The listing builds one solid part. Answer for the finished solid, in the listing's coordinates (mm). Face numbers are marked on the shaded views. A direction names the side the tool comes from. Coordinates: 2 decimals unless noted, no trailing zeros. Write each loop counter-clockwise with the first axis right and the second up, starting at its lowest first coordinate (ties: lowest second). Pieces come first, ordered by that corner, then holes.
(1) The part is cut by section C-C on y = 14.5. Determine the outline of the cut face in (x, z), plus the area to 3 significant figures.
(2) The part is cut by section A-A on z = 25. Determine the outline of the cut face in (x, y).
(3) The part is cut by section D-D on z = 17.5. Determine the outline of the cut face in (x, y).
(4) For a pull along Y with two mould halves and no side action, classify the marked faces 6, 7, 8 and 9 as +Y half, -Y half, draft (parallel to the pull), parting line (faces both ways), or undercut.
(5) The part is cut by section B-B on x = 7. Determine the outline of the cut face in (y, z).
(6) Given P1, Ø2.5, axis at x = 39.57, z = 25, coming from the +Y side; P2, Ø7.5, axis at y = -26.5, z = 4, coming from the +X side; P3, Ø3, axis at x = 3, y = -28, coming from the +Z side; P4, Ø3, axis at y = -7.5, z = 24.5, coming from the -X side, each flat-ended and moving along its own axis, determine where each tip first touches the part or whether it passes through.
(7) Which of the six approach directions +Z, -Z, +X, -X, +Y, -Y give full straight-line access (tool end or side, diameter ignored) to the marked faces 1, 2, 3, 4 and 5?
(8) Straight lines are drawn through the part: line 1 (X direction, y = -5, z = 25); line 2 (Y direction, x = 39, z = 11); line 3 (X direction, y = -7, z = 17). For each, find the intervals that lie inside material, in ascending order.
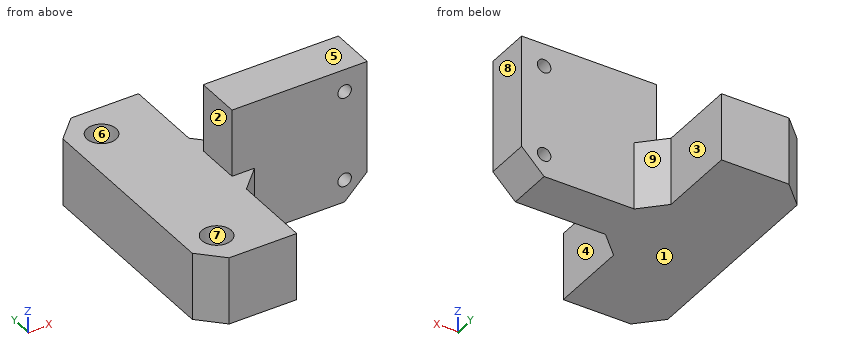
Autodesk Inventor part; units mm, degrees
ref_plane "YZ Plane" through (0, 0, 0) normal (1, 0, 0) x (0, 1, 0)
ref_plane "XZ Plane" through (0, 0, 0) normal (0, 1, 0) x (-1, 0, 0)
ref_plane "XY Plane" through (0, 0, 0) normal (0, 0, 1) x (1, 0, 0)
sketch "Sketch1" plane through (0, 0, 0) normal (0, 0, 1) x (1, 0, 0)
  line L0 (-5.4307, 20.6828) -> (14.5693, 20.6828)
  line L1 (14.5693, 20.6828) -> (14.5693, -34.3172)
  line L2 (14.5693, -34.3172) -> (-5.4307, -34.3172)
  line L3 (-5.4307, -34.3172) -> (-5.4307, 20.6828)
  point P0 (0, 0)
  dimension "d0" = 55
  dimension "d1" = 20
extrude "Extrusion1" add sketch "Sketch1" along normal blind 15
sketch "Sketch2" plane through (0, 0, 15) normal (0, 0, 1) x (1, 0, 0)
  line L0 (14.5693, 20.6828) -> (-5.4307, 20.6828)
  line L1 (-5.4307, -34.3172) -> (-5.4307, 20.6828)
  line L2 (-5.4307, -34.3172) -> (14.5693, -34.3172)
  circle A0 centre (1.5693, 13.1828) radius 3.25
  circle A1 centre (1.5693, -26.8172) radius 3.25
  point P0 (0, 0)
  dimension "d4" = 40
  dimension "d5" = 7.5
  dimension "d6" = 7
  dimension "d7" = 7.5
  dimension "d8" = 6.5
  dimension "d9" = 6.5
extrude "Extrusion2" cut sketch "Sketch2" against normal blind 10
sketch "Sketch3" plane through (0, 0, 0) normal (0, 0, -1) x (-1, 0, 0)
  line L0 (-14.5693, -34.3172) -> (-14.5693, 20.6828)
  line L1 (-14.5693, -1.8172) -> (-44.5693, -1.8172)
  line L2 (-44.5693, -1.8172) -> (-44.5693, -11.8172)
  line L3 (-44.5693, -11.8172) -> (-14.5693, -11.8172)
  line L4 (-14.5693, -11.8172) -> (-14.5693, -1.8172)
  line L5 (5.4307, 20.6828) -> (5.4307, -34.3172)
  point P0 (0, 0)
  point P1 (5.4307, -6.8172)
  dimension "d12" = 10
  dimension "d13" = 5
  dimension "d14" = 30
extrude "Extrusion3" add sketch "Sketch3" against normal blind 30
sketch "Sketch4" plane through (14.5693, -1.8172, 0) normal (0, 1, 0) x (1, 0, 0)
  line L0 (30, 0) -> (0, 0)
  line L1 (30, 0) -> (30, -30)
  line L2 (30, -30) -> (0, -30)
  point P0 (-14.5693, 0)
  point P1 (25, -5)
  point P2 (25, -25)
  dimension "d17" = 5
  dimension "d18" = 5
  dimension "d19" = 5
  dimension "d20" = 5
hole "Hole1" at (39.5693, -1.8172, 5) at (39.5693, -1.8172, 25) direction (0, -1, 0) diameter 3 depth 10 tip angle 118
chamfer "Chamfer1" distance 5 angle 45 1 edges at (44.5693, -6.8172, 0)
chamfer "Chamfer2" distance 5 angle 45 2 edges at (14.5693, -1.8172, 7.5) (14.5693, -11.8172, 7.5)
chamfer "Chamfer3" distance 5 angle 45 2 edges at (-5.4307, -34.3172, 7.5) (-5.4307, 20.6828, 7.5)
properties part number "Col support top"
Model answer:
1. outline: (-5.43, 0) - (14.57, 0) - (14.57, 15) - (4.54, 15) - (4.54, 5) - (-1.4, 5) - (-1.4, 15) - (-5.43, 15) - close
1. area: 241 mm2
2. outline: (14.57, -11.82) - (38.07, -11.82) - (38.07, -1.82) - (14.57, -1.82) - close; (41.07, -11.82) - (44.57, -11.82) - (44.57, -1.82) - (41.07, -1.82) - close
3. outline: (14.57, -11.82) - (44.57, -11.82) - (44.57, -1.82) - (14.57, -1.82) - close
4. face 6: undercut
4. face 7: undercut
4. face 8: draft
4. face 9: +Y half
5. outline: (-34.32, 0) - (20.68, 0) - (20.68, 15) - (-34.32, 15) - close
6. P1: passes through
6. P2: stops at x = 14.57
6. P3: stops at z = 15
6. P4: stops at x = 14.57
7. face 1: -Z, +X, -X, +Y, -Y
7. face 2: +Z, -X, +Y, -Y
7. face 3: +Z, -Z, +X, +Y
7. face 4: +Z, -Z, +X, -Y
7. face 5: +Z, +X, -X, +Y, -Y
8. line 1: x = 14.57 to 38.07, 41.07 to 44.57
8. line 2: y = -11.82 to -1.82
8. line 3: x = 14.57 to 44.57
